Source: three-view drawing plus pictorial views. Frame: mm from the lowest corner of the part. A direction names the side the tool comes from. Round coordinates to 2 decimals unless told otherwise and drop trailing zeros. Loops run counter-clockwise (first coordinate to the right, second up) from the corner with the lowest first, then second, coordinate; pieces in that order, holes last. Notation, with made-up numbers: (17, 53) -> (39, 53) arc R15 ccw to (39, 67) -> close; hole circle Ø8 at (36.5, 67). An arc over 180 degrees is marked (long way). Answer in a Markdown table with one row per item. Add a question column.
Q1. Pin query (flat end, axial travel): pin 1 (6 mm diameter, centred on x = 11.5, z = 8, fed in from -Y); pin 2 (0.6 mm diameter, centred on x = 5, y = 5, fed in from -Z); pin 3 (6 mm diameter, centred on x = 18.5, y = 7, fed in from +Z). Return the tip coordinate at first contact, or that it passes through.
Q2. Reachability of the marked faces 1, 2, 3 and 4 from +Z, -Z, +X, -X, +Y, -Y: full face, straight path, thin tool, end or side. Return the list, or none.
Q3. Section A-A, the plane z = 3.75. Output: boundary loops of the cut face in (x, y), and give its area (3 significant figures).
Q4. Ray query, L1, parallel to Y at x = 7, z = 0.15; L2, parallel to Y at x = 15.5, z = 3.75; L3, parallel to Y at x = 9, z = 0.3. Return the intervals inside material, ascending. Write a range as from..to.
Q5. Section C-C, the plane y = 3.5. Output: boundary loops of the cut face in (x, z).
Q6. Section D-D, the plane x = 17. Output: boundary loops of the cut face in (y, z).
Q7. Section B-B, the plane x = 7. Output: boundary loops of the cut face in (y, z).
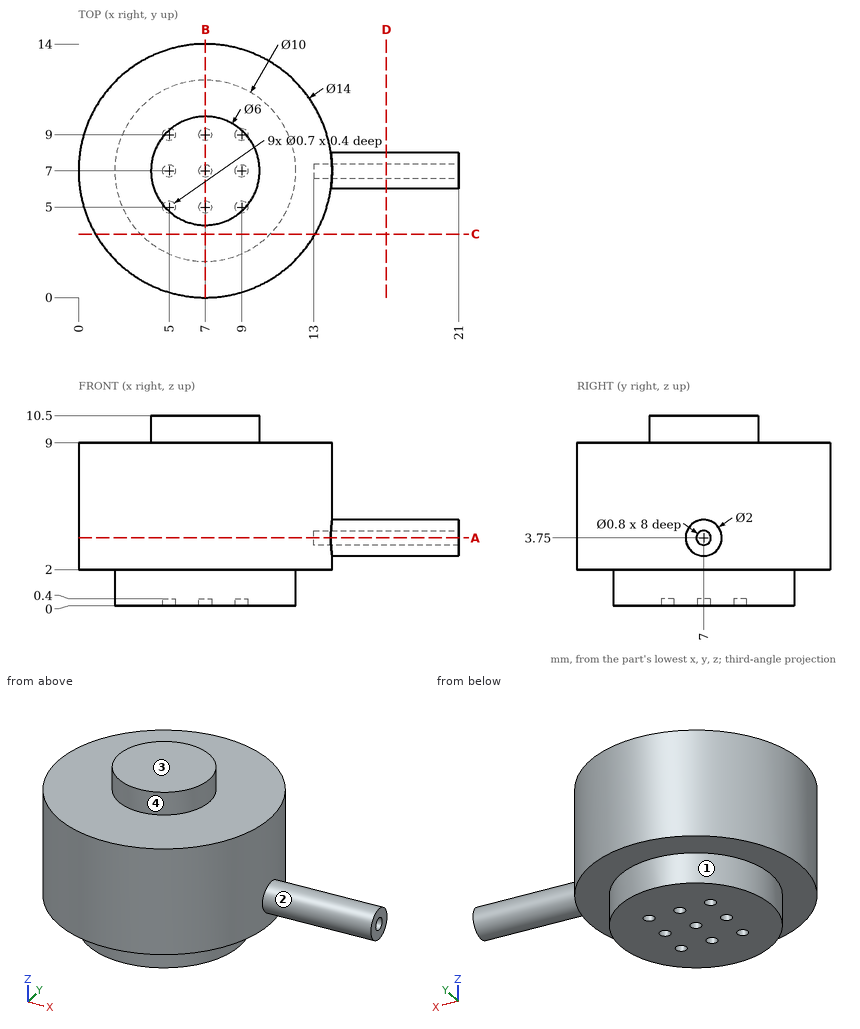
Answer block:
| question | item | result |
|---|---|---|
| 1 | pin 1 | y = 0.16 |
| 1 | pin 2 | z = 0.4 |
| 1 | pin 3 | z = 4.75 |
| 2 | face 1 | -Z |
| 2 | face 2 | +X |
| 2 | face 3 | +Z, +X, -X, +Y, -Y |
| 2 | face 4 | +Z |
| 3 | outline | (13, 6.6) -> (13, 7.4) -> (21, 7.4) -> (21, 8) -> (13.93, 8) arc R7 ccw (long way) to (13.93, 6) -> (21, 6) -> (21, 6.6) -> close |
| 3 | area | 162 mm^2 |
| 4 | L1 | 2..4.65, 5.35..6.65, 7.35..8.65, 9.35..12 |
| 4 | L2 | 6..6.6, 7.4..8 |
| 4 | L3 | 2.42..4.65, 5.35..6.65, 7.35..8.65, 9.35..11.58 |
| 5 | outline | (0.94, 2) -> (3.43, 2) -> (3.43, 0) -> (10.57, 0) -> (10.57, 2) -> (13.06, 2) -> (13.06, 9) -> (0.94, 9) -> close |
| 6 | outline | circle Ø2 at (7, 3.75); hole circle Ø0.8 at (7, 3.75) |
| 7 | outline | (0, 2) -> (2, 2) -> (2, 0) -> (4.65, 0) -> (4.65, 0.4) -> (5.35, 0.4) -> (5.35, 0) -> (6.65, 0) -> (6.65, 0.4) -> (7.35, 0.4) -> (7.35, 0) -> (8.65, 0) -> (8.65, 0.4) -> (9.35, 0.4) -> (9.35, 0) -> (12, 0) -> (12, 2) -> (14, 2) -> (14, 9) -> (10, 9) -> (10, 10.5) -> (4, 10.5) -> (4, 9) -> (0, 9) -> close |
